Verification items for this drawing (mm, ordinates from the low corner). A direction names the side the tool comes from. Round coordinates to 2 decimals unless told otherwise and drop trailing zeros. Order: outer loops, then holes, each group sorted by start corner. A loop starts at its lowest first (then second) coordinate and runs counter-clockwise, first axis right, second up.
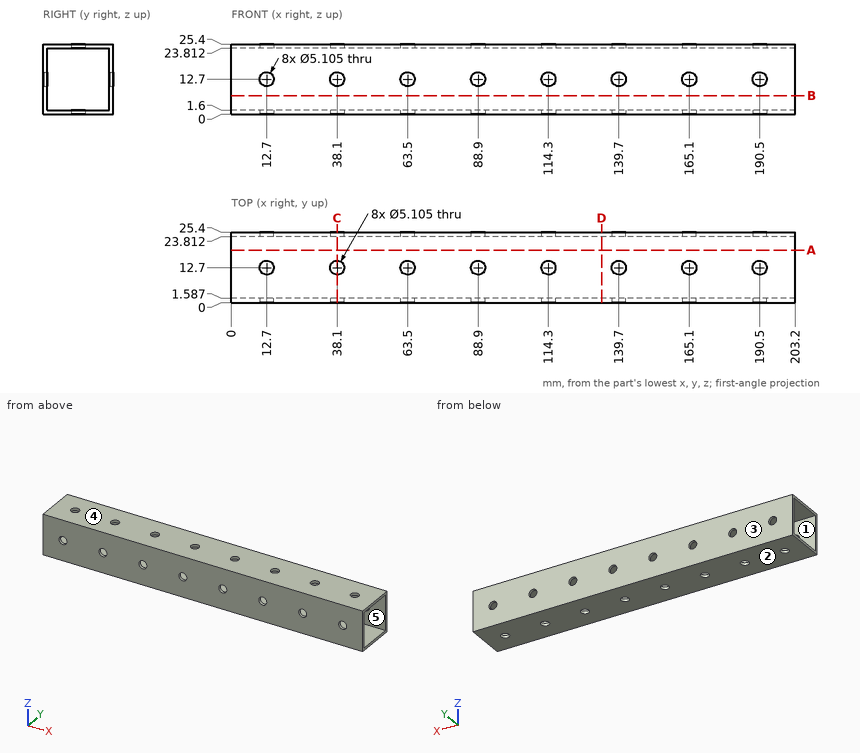
Item 1: Release check for a two-part mould opening along Y. For the marked faces 3, 4 and 5 record: released by +Y, released by -Y, zero draft, split by the parting line, or undercut.
Answer:
face 3: released by +Y
face 4: zero draft
face 5: undercut
Item 2: Access from +Z, -Z, +X, -X, +Y, -Y to the whole of each face (thin tool, end or side, straight path). Record for the marked faces 1 and 2.
Answer:
face 1: +X, -X
face 2: -Z, +X, -X, +Y, -Y
Item 3: Scan lines: line 1 along Y through (x, z) = (90, 7); line 2 along Z through (x, y) = (114, 7.75); line 3 along Z through (x, y) = (190.5, 24.5). Record each from-to range of solid material in increasing order.
Answer:
line 1: y = 0 to 1.59, 23.81 to 25.4
line 2: z = 0 to 1.6, 23.81 to 25.4
line 3: z = 0 to 10.15, 15.25 to 25.4
Item 4: Sectioned sample at A-A (y = 19). Record the cut outline in (x, z).
Answer:
outline: (0, 0) - (203.2, 0) - (203.2, 1.6) - (0, 1.6) - close; (0, 23.81) - (203.2, 23.81) - (203.2, 25.4) - (0, 25.4) - close
Item 5: Sectioned sample at C-C (x = 38.1). Record the cut outline in (y, z).
Answer:
outline: (0, 0) - (10.15, 0) - (10.15, 1.6) - (1.59, 1.6) - (1.59, 10.15) - (0, 10.15) - close; (0, 15.25) - (1.59, 15.25) - (1.59, 23.81) - (10.15, 23.81) - (10.15, 25.4) - (0, 25.4) - close; (15.25, 0) - (25.4, 0) - (25.4, 10.15) - (23.81, 10.15) - (23.81, 1.6) - (15.25, 1.6) - close; (15.25, 23.81) - (23.81, 23.81) - (23.81, 15.25) - (25.4, 15.25) - (25.4, 25.4) - (15.25, 25.4) - close
Item 6: Sectioned sample at D-D (x = 133.5). Record the cut outline in (y, z).
Answer:
outline: (0, 0) - (25.4, 0) - (25.4, 25.4) - (0, 25.4) - close; hole (1.59, 1.6) - (23.81, 1.6) - (23.81, 23.81) - (1.59, 23.81) - close
Item 7: Sectioned sample at B-B (z = 6.75). Record the cut outline in (x, y).
Answer:
outline: (0, 0) - (203.2, 0) - (203.2, 1.59) - (0, 1.59) - close; (0, 23.81) - (203.2, 23.81) - (203.2, 25.4) - (0, 25.4) - close
